Design review of the part built by this model. Coordinates are the model's own, in mm. A direction names the side the tool comes from. Coordinates: 2 decimals unless noted, no trailing zeros. Loops run counter-clockwise (first coordinate to the right, second up) from the corner with the lowest first, then second, coordinate; pieces in that order, holes last. Notation, with made-up numbers: M 30,84 L 45,84 A24 ccw 45,121 Z; hole C 55.5,38 d8. An arc over 180 degrees is marked long. One line per item, written item: value.
Autodesk Inventor part; units mm, degrees
ref_plane "YZ Plane" through (0, 0, 0) normal (1, 0, 0) x (0, 1, 0)
ref_plane "XZ Plane" through (0, 0, 0) normal (0, 1, 0) x (-1, 0, 0)
ref_plane "XY Plane" through (0, 0, 0) normal (0, 0, 1) x (1, 0, 0)
sketch "Sketch1" plane through (0, 0, 0) normal (0, 1, 0) x (-1, 0, 0)
  line L0 (2.286, 0) -> (10.414, 0)
  line L1 (12.7, -2.286) -> (12.7, -10.414)
  line L2 (10.414, -12.7) -> (2.286, -12.7)
  line L3 (0, -10.414) -> (0, -2.286)
  line L4 (8.1534, -4.0386) -> (4.5466, -4.0386)
  line L5 (4.0386, -4.5466) -> (4.0386, -8.1534)
  line L6 (4.5466, -8.6614) -> (8.1534, -8.6614)
  line L7 (8.6614, -8.1534) -> (8.6614, -4.5466)
  line L8 (10.414, 0) -> (12.7, -2.286)
  line L9 (12.7, -10.414) -> (10.414, -12.7)
  line L10 (2.286, -12.7) -> (0, -10.414)
  line L11 (2.286, 0) -> (0, -2.286)
  arc A0 (8.6614, -4.5466) -> (8.1534, -4.0386) centre (8.1534, -4.5466) ccw
  arc A1 (8.1534, -8.6614) -> (8.6614, -8.1534) centre (8.1534, -8.1534) ccw
  arc A2 (4.0386, -8.1534) -> (4.5466, -8.6614) centre (4.5466, -8.1534) ccw
  arc A3 (4.5466, -4.0386) -> (4.0386, -4.5466) centre (4.5466, -4.5466) ccw
  line L12 (8.1534, -4.5466) -> (4.5466, -8.1534) construction
  line L13 (12.7, -10.414) -> (0, -2.286) construction
  point P0 (0, 0)
  point P1 (12.7, -12.7)
  point P2 (12.7, 0)
  point P3 (0, -12.7)
  point P4 (4.0386, -8.6614)
  point P5 (8.6614, -8.6614)
  point P6 (6.35, -6.35)
  dimension "d1" = 12.7
  dimension "d2" = 4.6228
  dimension "d3" = 2.286
  dimension "d4" = 2.286
  dimension "d5" = 2.286
  dimension "d6" = 2.286
  dimension "d7" = 2.286
  dimension "d8" = 2.286
  dimension "d9" = 2.286
  dimension "d10" = 2.286
  dimension "d11" = 0.508
extrude "Body" add sketch "Sketch1" along normal blind 1.5875
sketch "Sketch2" plane through (0, 1.5875, 0) normal (0, 1, 0) x (1, 0, 0)
  arc A0 (-8.1534, 8.6614) -> (-8.6614, 8.1534) centre (-8.1534, 8.1534) ccw construction
  arc A1 (-4.5466, 4.0386) -> (-4.0386, 4.5466) centre (-4.5466, 4.5466) ccw construction
  circle A2 centre (-6.35, 6.35) radius 2.1844
  line L0 (-8.1534, 8.1534) -> (-4.5466, 4.5466) construction
  point P0 (0, 0)
  dimension "d14" = 4.3688
surface extrude "Circle" sketch "Sketch2" against normal up to surface (1.5875 mm away) shown yes curves A2
pattern_linear "Rectangular Pattern1" count 3 spacing 12.7 along (0, 0, -1) of "Body", "Circle"
equation "\"d22\" = d19"
(1) Mouldability with a two-part tool opening along X and no side actions: class faces 1 (the flat face through (-1.159, 0.783, -13.827)), 2 (the flat face through (-11.541, 0.783, -13.827)), 3 (the flat face through (-8.661, 1, -19)) as released by +X, released by -X, zero draft, split by the parting line, or undercut.
Reply:
face 1: released by +X
face 2: released by -X
face 3: undercut
(2) We need section B-B on x = -7. State the section outline as (y, z) points, then the cut area to 3 significant figures.
Reply:
outline: M 0,-38.1 L 1.59,-38.1 L 1.59,-34.06 L 0,-34.06 Z; M 0,-29.44 L 1.59,-29.44 L 1.59,-21.36 L 0,-21.36 Z; M 0,-16.74 L 1.59,-16.74 L 1.59,-8.66 L 0,-8.66 Z; M 0,-4.04 L 1.59,-4.04 L 1.59,0 L 0,0 Z
area: 38.5 mm2
(3) We need section A-A on z = -19. State the section outline as (x, y) points.
Reply:
outline: M -12.7,0 L -8.66,0 L -8.66,1.59 L -12.7,1.59 Z; M -4.04,0 L 0,0 L 0,1.59 L -4.04,1.59 Z
(4) Tool access review of faces 4 (the flat face through (-1.159, 0.783, -24.273)), 5 (the flat face through (-8.661, 1, -6)), 6 (the flat face through (-11.573, 0.783, -11.541)): name each direction out of +Z, -Z, +X, -X, +Y, -Y from which nothing blocks a thin tool from reaching the whole face with its end or side.
Reply:
face 4: +X, +Y, -Y
face 5: +Y, -Y
face 6: -X, +Y, -Y
(5) We need section C-C on y = 1. State how many separate pieces and enclosed holes the cut face has, then the cut area to 3 significant figures.
Reply:
separate pieces: 1
enclosed holes: 3
area: 389 mm2
(6) We need section D-D on x = -1.5. State the section outline as (y, z) points.
Reply:
outline: M 0,-37.31 L 1.59,-37.31 L 1.59,-26.19 L 0,-26.19 Z; M 0,-24.61 L 1.59,-24.61 L 1.59,-13.49 L 0,-13.49 Z; M 0,-11.91 L 1.59,-11.91 L 1.59,-0.79 L 0,-0.79 Z
(7) To check wall thickness, follow line 1 along Z through (x, y) = (-6.5, 1.35); line 2 along X through (y, z) = (0.3, -31); line 3 along Z through (x, y) = (-12, 1.25). State the ranges of each line that lie inside material, in increasing order. Write a range as [from, to].
Reply:
line 1: z = [-38.1, -34.06], [-29.44, -21.36], [-16.74, -8.66], [-4.04, 0]
line 2: x = [-12.7, -8.66], [-4.04, 0]
line 3: z = [-36.51, -26.99], [-23.81, -14.29], [-11.11, -1.59]
